```python
from build123d import *

# Parameters (mm, degrees)
F0_W     = 102
F0_H     = 27.1
F1_DEPTH = 1
F2_W     = 90
F2_H     = 1.5
F3_DEPTH = 1


# Not quite as in the source:
# - a feature names something its author has since deleted; it is built from what else it names


with BuildPart() as f1:
    # F0 (on Top) → F1 (new body)
    with BuildSketch(Plane.XY):
        with Locations((-1, -1)):
            Rectangle(F0_W, F0_H)
    extrude(amount=F1_DEPTH)

    # F2 (on face) → F3 (join)
    with BuildSketch(Plane.XY.offset(1)):
        Polygon((-42.2541592645, 8.3261114968), (-41.0671610971, 8.7179473687), (-40.8130018326, 9.9418358719), (-41.7458407355, 10.7738885032), (-42.9328389029, 10.3820526313), (-43.1869981674, 9.1581641281), align=None)
        Polygon((-13.0671610971, 8.7179473687), (-12.8130018326, 9.9418358719), (-13.7458407355, 10.7738885032), (-14.9328389029, 10.3820526313), (-15.1869981674, 9.1581641281), (-14.2541592645, 8.3261114968), align=None)
        Polygon((14.9328389029, 8.7179473687), (15.1869981674, 9.9418358719), (14.2541592645, 10.7738885032), (13.0671610971, 10.3820526313), (12.8130018326, 9.1581641281), (13.7458407355, 8.3261114968), align=None)
        Polygon((42.9328389029, 8.7179473687), (43.1869981674, 9.9418358719), (42.2541592645, 10.7738885032), (41.0671610971, 10.3820526313), (40.8130018326, 9.1581641281), (41.7458407355, 8.3261114968), align=None)
        Polygon((-43.1869981674, -9.1581641281), (-42.9328389029, -10.3820526313), (-41.7458407355, -10.7738885032), (-40.8130018326, -9.9418358719), (-41.0671610971, -8.7179473687), (-42.2541592645, -8.3261114968), align=None)
        Polygon((-14.2541592645, -8.3261114968), (-15.1869981674, -9.1581641281), (-14.9328389029, -10.3820526313), (-13.7458407355, -10.7738885032), (-12.8130018326, -9.9418358719), (-13.0671610971, -8.7179473687), align=None)
        Polygon((13.7458407355, -8.3261114968), (12.8130018326, -9.1581641281), (13.0671610971, -10.3820526313), (14.2541592645, -10.7738885032), (15.1869981674, -9.9418358719), (14.9328389029, -8.7179473687), align=None)
        Polygon((42.9328389029, -8.7179473687), (41.7458407355, -8.3261114968), (40.8130018326, -9.1581641281), (41.0671610971, -10.3820526313), (42.2541592645, -10.7738885032), (43.1869981674, -9.9418358719), align=None)
        with Locations((-0.065032054, 3.9994713191)):
            Rectangle(F2_W, F2_H)
        Rectangle(F2_W, F2_H)
        with Locations((0, -4)):
            Rectangle(F2_W, F2_H)
    extrude(amount=F3_DEPTH)


solid = f1.part
```
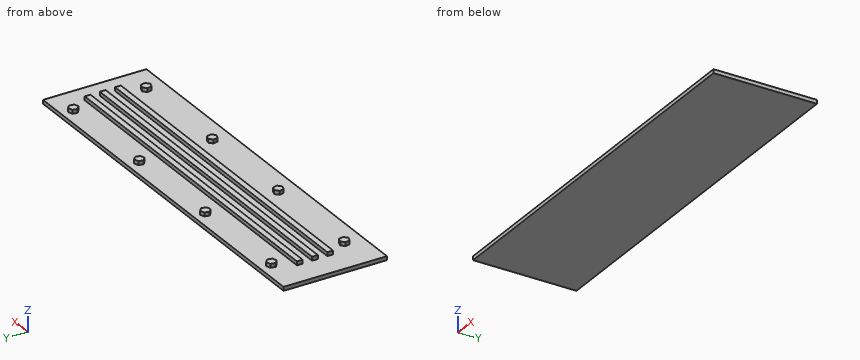
Part model, mm, in its own coordinate system. Round coordinates to 2 decimals unless told otherwise and drop trailing zeros. Loops run counter-clockwise (first coordinate to the right, second up) from the corner with the lowest first, then second, coordinate; pieces in that order, holes last.
Item 1: Cut at A-A, the plane x = 18.5. Give the cut face in (y, z).
Item 2: Drop a flat-ended pin along its axis: P1, Ø0.5, axis at x = -16.5, z = 1.5, coming from the +Y side. Give the stop position or say it passes through.
Item 3: Drill centre lines: line 1 (Y direction, x = -9, z = 1.5); line 2 (X direction, y = 8.75, z = 1.6); line 3 (X direction, y = 9, z = 1.6). Where is each one in solid material? Low to high.
Item 4: Cut at B-B, the plane z = 1.55. State how many separate pieces and enclosed holes the cut face has, then the cut area to 3 significant figures.
Item 5: Cut at C-C, the plane y = 1.75. Give the cut face in (x, z).
A:
1. outline: (-14.55, 0) - (12.55, 0) - (12.55, 1) - (4.75, 1) - (4.75, 2) - (3.25, 2) - (3.25, 1) - (0.75, 1) - (0.75, 2) - (-0.75, 2) - (-0.75, 1) - (-3.25, 1) - (-3.25, 2) - (-4.75, 2) - (-4.75, 1) - (-14.55, 1) - close
2. P1: stops at y = 4.75
3. line 1: y = -4.75 to -3.25, -0.75 to 0.75, 3.25 to 4.75
3. line 2: x = -42.73 to -41.06, -14.73 to -13.06, 13.27 to 14.94, 41.27 to 42.94
3. line 3: x = -43.01 to -41.01, -15.01 to -13.01, 12.99 to 14.99, 40.99 to 42.99
4. separate pieces: 11
4. enclosed holes: 0
4. area: 437 mm2
5. outline: (-52, 0) - (50, 0) - (50, 1) - (-52, 1) - close
